CAD build for the part. Positions are in the model's coordinates, mm. A direction names the side the tool comes from. Round coordinates to 2 decimals unless told otherwise and drop trailing zeros. Write each loop counter-clockwise with the first axis right and the second up, starting at its lowest first coordinate (ties: lowest second). Pieces come first, ordered by that corner, then holes. Notation, with made-up numbers: (74, 24) -> (131, 24) arc R11 cw to (131, 34) -> close; hole circle Ø4 at (-10, -21). An arc over 180 degrees is marked (long way). Answer in a Markdown table with one row per item. Add a question column.
```python
from build123d import *

# Parameters (mm, degrees)
SKIZZE1_R                            = 2.35
AUFSATZ_LINEAR_AUSTRAGEN1_DEPTH      = 12
AUFSATZ_LINEAR_AUSTRAGEN1_2_DEPTH    = 12
AUFSATZ_LINEAR_AUSTRAGEN1_3_DEPTH    = 12
AUFSATZ_LINEAR_AUSTRAGEN1_4_DEPTH    = 12
AUFSATZ_LINEAR_AUSTRAGEN1_5_DEPTH    = 12
SKIZZE1_3_R                          = 2.35
AUFSATZ_LINEAR_AUSTRAGEN4_DEPTH      = 9.5
SKIZZE2_R                            = 3.25
AUFSATZ_LINEAR_AUSTRAGEN2_DEPTH      = 1
AUFSATZ_LINEAR_AUSTRAGEN3_DEPTH      = 1
SKIZZE5_R                            = 2.6
AUFSATZ_LINEAR_AUSTRAGEN5_DEPTH      = 4.5
FASE1_SIZE                           = 0.5
FASE2_SIZE                           = 0.5
FASE3_SIZE                           = 0.5
SCHNITT_LINEAR_AUSTRAGEN1_DEPTH      = 7
SCHNITT_LINEAR_AUSTRAGEN1_DEPTH_BACK = 27.592507318
VERRUNDUNG1_R                        = 1


with BuildPart() as part:
    # Skizze1 → Aufsatz-Linear austragen1 (new body)
    with BuildSketch(Plane.XY):
        with Locations((-17.068817434, 1.838554139)):
            Circle(SKIZZE1_R)
    extrude(amount=AUFSATZ_LINEAR_AUSTRAGEN1_DEPTH)



with BuildPart() as body_2:
    # Skizze1 → Aufsatz-Linear austragen1 2 (new body)
    with BuildSketch(Plane.XY):
        with Locations((-9.321817434, 1.838554139)):
            Circle(SKIZZE1_R)
    extrude(amount=AUFSATZ_LINEAR_AUSTRAGEN1_2_DEPTH)


with BuildPart() as body_3:
    # Skizze1 → Aufsatz-Linear austragen1 3 (new body)
    with BuildSketch(Plane.XY):
        Circle(SKIZZE1_R)
    extrude(amount=AUFSATZ_LINEAR_AUSTRAGEN1_3_DEPTH)


with BuildPart() as body_4:
    # Skizze1 → Aufsatz-Linear austragen1 4 (new body)
    with BuildSketch(Plane.XY):
        with Locations((0.007570249, 6.993531953)):
            Circle(SKIZZE1_R)
    extrude(amount=AUFSATZ_LINEAR_AUSTRAGEN1_4_DEPTH)


with BuildPart() as body_5:
    # Skizze1 → Aufsatz-Linear austragen1 5 (new body)
    with BuildSketch(Plane.XY):
        with Locations((8.839182566, 1.838554139)):
            Circle(SKIZZE1_R)
    extrude(amount=AUFSATZ_LINEAR_AUSTRAGEN1_5_DEPTH)


with BuildPart() as body_6:
    # Skizze1<3> → Aufsatz-Linear austragen4 (new body)
    with BuildSketch(Plane.XY):
        with Locations((16.586182566, 1.838554139)):
            Circle(SKIZZE1_3_R)
    extrude(amount=AUFSATZ_LINEAR_AUSTRAGEN4_DEPTH)


with BuildPart() as part_1:
    add(part.part)

    add(body_2.part)  # Aufsatz-Linear austragen2 merges body 2

    add(body_3.part)  # Aufsatz-Linear austragen2 merges body 3

    add(body_4.part)  # Aufsatz-Linear austragen2 merges body 4

    add(body_5.part)  # Aufsatz-Linear austragen2 merges body 5

    add(body_6.part)  # Aufsatz-Linear austragen2 merges body 6
    # Skizze2 → Aufsatz-Linear austragen2 (add)
    with BuildSketch(Plane.XY):
        with Locations((-17.068817434, 1.838554139)):
            Circle(SKIZZE2_R)
        with Locations((-9.321817434, 1.838554139)):
            Circle(SKIZZE2_R)
        Circle(SKIZZE2_R)
        with Locations((0.007570249, 6.993531953)):
            Circle(SKIZZE2_R)
        with Locations((8.839182566, 1.838554139)):
            Circle(SKIZZE2_R)
        with Locations((16.586182566, 1.838554139)):
            Circle(SKIZZE2_R)
    extrude(amount=AUFSATZ_LINEAR_AUSTRAGEN2_DEPTH)

    # Skizze3 → Aufsatz-Linear austragen3 (add)
    with BuildSketch(Plane.XY):
        Polygon((-18.068817434, 13.164615586), (-18.068817434, 4.930883358), (-16.068817434, 4.930883358), (-16.068817434, 11.164615586), (-10.321817434, 11.164615586), (-10.321817434, 4.930883358), (-8.321817434, 4.930883358), (-8.321817434, 11.164615586), (-5.921817434, 11.164615586), (-5.921817434, 5.993531953), (-3.08475897, 5.993531953), (-3.08475897, 7.993531953), (-3.921817434, 7.993531953), (-3.921817434, 11.164615586), (3.439182566, 11.164615586), (3.439182566, 1), (3.092329219, 1), (3.092329219, -1), (3.439182566, -1), (5.439182566, -1), (5.439182566, 1), (5.439182566, 11.164615586), (7.839182566, 11.164615586), (7.839182566, 4.930883358), (9.839182566, 4.930883358), (9.839182566, 11.164615586), (15.586182566, 11.164615586), (15.586182566, 4.930883358), (17.586182566, 4.930883358), (17.586182566, 13.164615586), align=None)
    extrude(amount=AUFSATZ_LINEAR_AUSTRAGEN3_DEPTH)

    # Skizze5 → Aufsatz-Linear austragen5 (add)
    with BuildSketch(Plane.XY.offset(1)):
        with Locations((-17.068817434, 1.838554139)):
            Circle(SKIZZE5_R)
        with Locations((-9.321817434, 1.838554139)):
            Circle(SKIZZE5_R)
        with Locations((0.007570249, 6.993531953)):
            Circle(SKIZZE5_R)
        Circle(SKIZZE5_R)
        with Locations((8.839182566, 1.838554139)):
            Circle(SKIZZE5_R)
        with Locations((16.586182566, 1.838554139)):
            Circle(SKIZZE5_R)
    extrude(amount=AUFSATZ_LINEAR_AUSTRAGEN5_DEPTH)

    # Fase1
    fase1_edges = [part_1.edges().sort_by_distance(p)[0] for p in [
        (-19.418817434, 1.838554139, 12),
        (-2.35, 0, 12),
        (-2.342429751, 6.993531953, 12),
        (6.489182566, 1.838554139, 12),
        (-11.671817434, 1.838554139, 12),
    ]]
    chamfer(fase1_edges, length=FASE1_SIZE)

    # Fase2
    fase2_edges = [part_1.edges().sort_by_distance(p)[0] for p in [
        (-19.668817434, 1.838554139, 1),
        (-11.921817434, 1.838554139, 1),
        (-2.592429751, 6.993531953, 1),
        (-2.6, 0, 1),
        (6.239182566, 1.838554139, 1),
        (13.986182566, 1.838554139, 1),
    ]]
    chamfer(fase2_edges, length=FASE2_SIZE)

    # Fase3
    fase3_edges = [part_1.edges().sort_by_distance(p)[0] for p in [
        (14.236182566, 1.838554139, 9.5),
    ]]
    chamfer(fase3_edges, length=FASE3_SIZE)

    # Skizze6 → Schnitt-Linear austragen1 (cut, two sides: drawn at the far end of the back side and taken through both)
    with BuildSketch(Plane.XY.offset(1).offset(-SCHNITT_LINEAR_AUSTRAGEN1_DEPTH_BACK)):
        with BuildLine():
            Line((2.789182566, 9.801413918), (2.789182566, 4.443241997))
            Line((2.789182566, 4.443241997), (3.439182566, 4.443241997))
            ThreePointArc((3.439182566, 4.443241997), (3.764166783, 7.122327957), (3.439182566, 9.801413918))
            Line((3.439182566, 9.801413918), (2.789182566, 9.801413918))
        make_face()
        with BuildLine():
            Line((6.089182566, 4.189181846), (6.089182566, -0.607667928))
            Line((6.089182566, -0.607667928), (5.439182566, -0.607667928))
            ThreePointArc((5.439182566, -0.607667928), (5.136833773, 1.790756959), (5.439182566, 4.189181846))
            Line((5.439182566, 4.189181846), (6.089182566, 4.189181846))
        make_face()
    extrude(amount=SCHNITT_LINEAR_AUSTRAGEN1_DEPTH + SCHNITT_LINEAR_AUSTRAGEN1_DEPTH_BACK, mode=Mode.SUBTRACT)

    # Verrundung1
    # the kernel refuses this fillet: 1 mm, written as the material it adds along each edge
    with BuildSketch(Plane(origin=(3.439182566, 1, 0), x_dir=(-1, 0, 0), z_dir=(0, 0, 1))) as verrundung1_piece_1:
        with BuildLine():
            CenterArc((1, -0.757231437), VERRUNDUNG1_R, 130.779268334, 49.220731666)
            Line((0, -0.757231437), (-0.02, -0.757231437))
            Line((-0.02, -0.757231437), (-0.02, 0))
            Line((-0.02, 0), (0, 0.02))
            ThreePointArc((0, 0.02), (0.173426673, 0.02), (0.333790414, 0.015144629))
            Line((0.333790414, 0.015144629), (0.346853347, 0))
        make_face()
    extrude(amount=1)
    with BuildSketch(Plane(origin=(9.839182566, 11.164615586, 0), x_dir=(1, 0, 0), z_dir=(0, 0, 1)), Plane(origin=(7.839182566, 11.164615586, 0), x_dir=(0, -1, 0), z_dir=(0, 0, 1)), Plane(origin=(3.439182566, 11.164615586, 0), x_dir=(0, -1, 0), z_dir=(0, 0, 1)), Plane(origin=(5.439182566, 11.164615586, 0), x_dir=(1, 0, 0), z_dir=(0, 0, 1)), Plane(origin=(-10.321817434, 11.164615586, 0), x_dir=(0, -1, 0), z_dir=(0, 0, 1)), Plane(origin=(-8.321817434, 11.164615586, 0), x_dir=(1, 0, 0), z_dir=(0, 0, 1)), Plane(origin=(-3.921817434, 11.164615586, 0), x_dir=(1, 0, 0), z_dir=(0, 0, 1)), Plane(origin=(-5.921817434, 11.164615586, 0), x_dir=(0, -1, 0), z_dir=(0, 0, 1))) as verrundung1_piece_2:
        with BuildLine():
            CenterArc((VERRUNDUNG1_R, -VERRUNDUNG1_R), VERRUNDUNG1_R, 90, 90)
            Line((0, -VERRUNDUNG1_R), (-VERRUNDUNG1_R * 0.02, -VERRUNDUNG1_R))
            Line((-VERRUNDUNG1_R * 0.02, -VERRUNDUNG1_R), (-VERRUNDUNG1_R * 0.02, VERRUNDUNG1_R * 0.02))
            Line((-VERRUNDUNG1_R * 0.02, VERRUNDUNG1_R * 0.02), (VERRUNDUNG1_R, VERRUNDUNG1_R * 0.02))
            Line((VERRUNDUNG1_R, VERRUNDUNG1_R * 0.02), (VERRUNDUNG1_R, 0))
        make_face()
    extrude(amount=1)
    with BuildSketch(Plane(origin=(-3.921817434, 7.993531953, 0), x_dir=(0, 1, 0), z_dir=(0, 0, 1))) as verrundung1_piece_3:
        with BuildLine():
            CenterArc((0.986635726, -1), VERRUNDUNG1_R, 90, 80.622325088)
            Line((0, -0.837058464), (-0.019732715, -0.833799634))
            ThreePointArc((-0.019732715, -0.833799634), (-0.02, -0.418529232), (-0.02, 0))
            Line((-0.02, 0), (0, 0.02))
            Line((0, 0.02), (0.986635726, 0.02))
            Line((0.986635726, 0.02), (0.986635726, 0))
        make_face()
    extrude(amount=1)
    # the kernel refuses this fillet: 1 mm, written as the material it takes off along each edge
    with BuildSketch(Plane(origin=(5.439182566, -1, -1.985478044), x_dir=(0, 1, 0), z_dir=(0, 0, 1))) as verrundung1_2_piece_1:
        with BuildLine():
            CenterArc((1, 0.794191217), VERRUNDUNG1_R, 180, 52.578930711)
            Line((0, 0.794191217), (-0.02, 0.794191217))
            Line((-0.02, 0.794191217), (-0.02, 0))
            Line((-0.02, 0), (0, -0.02))
            ThreePointArc((0, -0.02), (0.196166036, -0.02), (0.380178714, -0.015883824))
            Line((0.380178714, -0.015883824), (0.392332072, 0))
        make_face()
    extrude(amount=4.970956087, mode=Mode.SUBTRACT)


solid = part_1.part
```
Item 1: Saw through at C-C on x = 0. Count the separate pieces of the cut face and the enclosed holes in it, then the cut area to 3 significant figures.
Item 2: Saw through at D-D on z = 6. Give the cut face in (x, y), then the cut area to 3 significant figures.
Item 3: Saw through at B-B on z = 4. Give the cut face in (x, y), then the cut area to 3 significant figures.
Item 4: Tool access for faces 1 (the flat face through (-18.069, 9.1, 0.5)), 2 (the cylindrical face through (-7.08, 2.54, 8.46)), 3 (the flat face through (-0.3, 11.165, 0.5)): list every direction of +Z, -Z, +X, -X, +Y, -Y with a clear straight run to the whole face (end or side of a thin tool).
Item 5: Drill centre lines: probe 1 along X at (y, z) = (-0.25, 8.25); probe 2 along X at (y, z) = (0, 8.25); probe 3 along X at (y, z) = (3, 0.75). Where is each one in solid material? Low to high.
Item 6: Pin check, flat tips, straight feed: pin 1 (1.5 mm diameter, centred on x = -13.5, z = 2, fed in from +Y); pin 2 (3 mm diameter, centred on x = 6, z = 9, fed in from -Y); pin 3 (3 mm diameter, centred on y = 5, z = 5, fed in from -X); pin 4 (0.8 mm diameter, centred on y = 9.5, z = 0.5, fed in from +X). Stop position of each tip, or through.
Item 7: Saw through at A-A on z = 11. Give the cut face in (x, y).
Recorded:
| question | item | result |
|---|---|---|
| 1 | separate pieces | 3 |
| 1 | enclosed holes | 0 |
| 1 | area | 123 mm2 |
| 2 | outline | circle Ø4.7 at (-17.07, 1.84); circle Ø4.7 at (-9.32, 1.84); circle Ø4.7 at (0, 0); circle Ø4.7 at (0.01, 6.99); circle Ø4.7 at (8.84, 1.84); circle Ø4.7 at (16.59, 1.84) |
| 2 | area | 104 mm2 |
| 3 | outline | circle Ø5.2 at (-17.07, 1.84); circle Ø5.2 at (-9.32, 1.84); circle Ø5.2 at (0, 0); circle Ø5.2 at (0.01, 6.99); circle Ø5.2 at (8.84, 1.84); circle Ø5.2 at (16.59, 1.84) |
| 3 | area | 127 mm2 |
| 4 | face 1 | +Z, -Z, -X, +Y |
| 4 | face 2 | +Z |
| 4 | face 3 | +Z, -Z |
| 5 | probe 1 | -18.15 to -15.99, -10.4 to -8.24, -2.34 to 2.34, 7.76 to 9.92, 15.51 to 17.66 |
| 5 | probe 2 | -18.53 to -15.61, -10.79 to -7.86, -2.35 to 2.35, 7.38 to 10.3, 15.12 to 18.05 |
| 5 | probe 3 | -20.1 to -14.03, -12.36 to -6.29, -1.25 to 1.25, 3.44 to 5.21, 6.09 to 11.87, 13.55 to 19.62 |
| 6 | pin 1 | through |
| 6 | pin 2 | y = -0.09 |
| 6 | pin 3 | x = -19.07 |
| 6 | pin 4 | x = 17.59 |
| 7 | outline | circle Ø4.7 at (-17.07, 1.84); circle Ø4.7 at (-9.32, 1.84); circle Ø4.7 at (0, 0); circle Ø4.7 at (0.01, 6.99); circle Ø4.7 at (8.84, 1.84) |
